```python
from build123d import *

# Parameters (mm, degrees)
BOSS_EXTRUDE1_DEPTH     = 150
BOSS_EXTRUDE2_DEPTH     = 150
SKETCH6_W               = 164.867200615
SKETCH6_H               = 10
BOSS_EXTRUDE4_DEPTH     = 107
BOSS_EXTRUDE5_DEPTH     = 10
BOSS_EXTRUDE6_DEPTH     = 10
SKETCH9_W               = 20
SKETCH9_H               = 170
SKETCH9_R               = 5
BOSS_EXTRUDE7_DEPTH     = 10
CUT_EXTRUDE2_DEPTH      = 281.132270411
CUT_EXTRUDE2_DEPTH_BACK = 281.132270411
CUT_EXTRUDE3_DEPTH      = 263.34809014
CUT_EXTRUDE3_DEPTH_BACK = 263.34809014


with BuildPart() as part:
    # Sketch2 → Boss-Extrude1 (new body)
    with BuildSketch(Plane.XY):
        Polygon((0, 0), (-97, 0), (-97, 107), (0, 10), align=None)
    extrude(amount=BOSS_EXTRUDE1_DEPTH)

    # Sketch4 → Boss-Extrude2 (add)
    with BuildSketch(Plane.XY.offset(150)):
        Polygon((-14.566399692, 24.566399692), (67.867200615, 107), (67.867200615, 0), (0, 0), (0, 10), align=None)
    extrude(amount=-BOSS_EXTRUDE2_DEPTH)

    # Sketch6 → Boss-Extrude4 (add)
    with BuildSketch(Plane(origin=(0, 0, 0), x_dir=(1, 0, 0), z_dir=(0, 1, 0))):
        with Locations((-14.566399692, -155)):
            Rectangle(SKETCH6_W, SKETCH6_H)
        with Locations((-14.566399692, 5)):
            Rectangle(SKETCH6_W, SKETCH6_H)
    extrude(amount=BOSS_EXTRUDE4_DEPTH)

    # Sketch7 → Boss-Extrude5 (add)
    with BuildSketch(Plane.XY.offset(160)):
        Polygon((-97, 107), (-14.566399692, 189.433600308), (67.867200615, 107), align=None)
    extrude(amount=-BOSS_EXTRUDE5_DEPTH)

    # Sketch8 → Boss-Extrude6 (add)
    with BuildSketch(Plane(origin=(0, 0, -10), x_dir=(-1, 0, 0), z_dir=(0, 0, -1))):
        Polygon((-67.867200615, 107), (97, 107), (14.566399692, 189.433600308), align=None)
    extrude(amount=-BOSS_EXTRUDE6_DEPTH)

    # Sketch9 → Boss-Extrude7 (add)
    # profile 1 of 2: a face of its own
    with BuildSketch(Plane(origin=(0, 0, 0), x_dir=(1, 0, 0), z_dir=(0, 1, 0))):
        with Locations((-107, -75)):
            Rectangle(SKETCH9_W, SKETCH9_H)
        with Locations(Location((-107, -145, 0), (0, 0, 270))):
            Circle(SKETCH9_R, mode=Mode.SUBTRACT)
        with Locations(Location((-107, -5, 0), (0, 0, 270))):
            Circle(SKETCH9_R, mode=Mode.SUBTRACT)
    # profile 2 of 2: a face of its own
    with BuildSketch(Plane(origin=(0, 0, 0), x_dir=(1, 0, 0), z_dir=(0, 1, 0))):
        with Locations((77.867200615, -75)):
            Rectangle(SKETCH9_W, SKETCH9_H)
        with Locations(Location((77.867200615, -145, 0), (0, 0, 90))):
            Circle(SKETCH9_R, mode=Mode.SUBTRACT)
        with Locations(Location((77.867200615, -5, 0), (0, 0, 90))):
            Circle(SKETCH9_R, mode=Mode.SUBTRACT)
    extrude(amount=BOSS_EXTRUDE7_DEPTH)

    # Sketch12 → Cut-Extrude2 (cut, two sides: drawn at the far end of the back side and taken through both)
    with BuildSketch(Plane.XY.offset(160).offset(-CUT_EXTRUDE2_DEPTH_BACK)):
        Polygon((-42.02, 161.98), (12.887200615, 161.98), (-14.566399692, 189.433600308), align=None)
    extrude(amount=CUT_EXTRUDE2_DEPTH + CUT_EXTRUDE2_DEPTH_BACK, mode=Mode.SUBTRACT)

    # Sketch14 → Cut-Extrude3 (cut, two sides: drawn at the far end of the back side and taken through both)
    with BuildSketch(Plane.XY.offset(160).offset(-CUT_EXTRUDE3_DEPTH_BACK)):
        Polygon((-14.566399692, 161.98), (67.867200615, 79.546399692), (67.867200615, 107), (12.887200615, 161.98), align=None)
    extrude(amount=CUT_EXTRUDE3_DEPTH + CUT_EXTRUDE3_DEPTH_BACK, mode=Mode.SUBTRACT)


solid = part.part
```
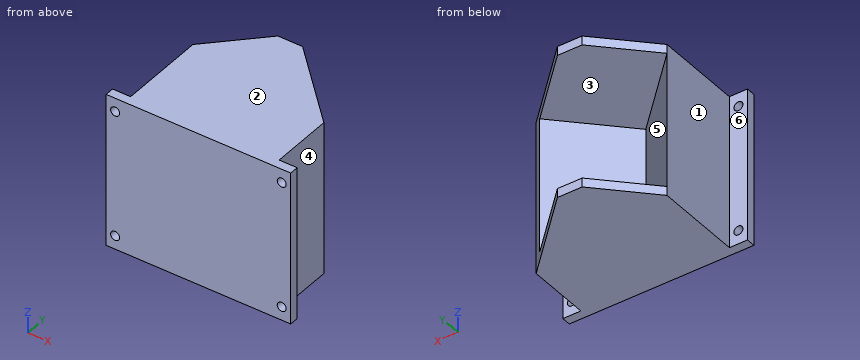
Can you work these out from the model? Positions are in its coordinate system, mm. Face numbers are marked on the shaded views. A direction names the side the tool comes from. Give positions to 0.01 mm unless a question says otherwise; leave off trailing zeros. Loops run counter-clockwise (first coordinate to the right, second up) from the corner with the lowest first, then second, coordinate; pieces in that order, holes last. Notation, with made-up numbers: M 53,45.5 L 64,45.5 A10 ccw 64,51.5 Z; hole C 80.5,-3 d1. An arc over 180 degrees is marked long. Answer in a Markdown table with one row per item.
1. Which directions (+Z, -Z, +X, -X, +Y, -Y) give clear straight access to the entire face, cutting with the end or side of a thin tool? Please do the marked faces 4, 5 and 6.
Taken from the geometry:
| item | result |
|---|---|
| face 4 | +Z, -Z, +X, +Y |
| face 5 | +Y |
| face 6 | +Z, -Z, -X, +Y |
2. Suppose I cut it at A-A on z = 5. Write out the boundary of the cut face in (x, y).
Taken from the geometry:
| item | result |
|---|---|
| outline | M -117,0 L -112,0 L -112,10 L -117,10 Z; M -102,0 L 72.87,0 L 72.87,10 L 67.87,10 L 67.87,79.55 L 54.14,93.27 L -14.57,24.57 L -97,107 L -97,10 L -102,10 Z; M 82.87,0 L 87.87,0 L 87.87,10 L 82.87,10 Z |
3. If I drill on line 1 along X through (y, z) = (6, 5); line 2 along Z through (x, y) = (-26.5, 101.5); line 3 along Y through (x, z) = (-101, 68), over which ranges is the centre line in solid material (lowest first)?
Taken from the geometry:
| item | result |
|---|---|
| line 1 | x = -117 to -112, -102 to 72.87, 82.87 to 87.87 |
| line 2 | z = -10 to 0, 150 to 160 |
| line 3 | y = 0 to 10 |
4. For pin 1 Ø5 at (x, z) = (-89.5, 25.5) entering from +Y; pin 2 Ø6 at (x, z) = (-105, 117.5) entering from +Y; pin 3 Ø3 at (y, z) = (22.5, 67) entering from -X; pin 4 Ø6 at (x, z) = (-107, 145) entering from -Y, each with a flat end and sliding along its axis, tell me the tip position at first contact or that it passes through.
Taken from the geometry:
| item | result |
|---|---|
| pin 1 | stops at y = 102 |
| pin 2 | stops at y = 10 |
| pin 3 | stops at x = -97 |
| pin 4 | passes through |
5. Suppose I cut it at D-D on z = 119. Write out the boundary of the cut face in (x, y).
Taken from the geometry:
| item | result |
|---|---|
| outline | M -117,0 L 87.87,0 L 87.87,10 L 67.87,10 L 67.87,79.55 L 54.14,93.27 L -14.57,24.57 L -97,107 L -97,10 L -117,10 Z |
6. Thinking about a two-plate mould opening in Z: for the marked faces 1, 2 and 3, which applies, released by +Z, released by -Z, zero draft, split by the parting line, or undercut?
Taken from the geometry:
| item | result |
|---|---|
| face 1 | zero draft |
| face 2 | released by +Z |
| face 3 | undercut |
7. Suppose I cut it at B-B on x = -107. Write out the boundary of the cut face in (y, z).
Taken from the geometry:
| item | result |
|---|---|
| outline | M 0,-10 L 10,-10 L 10,0 L 0,0 Z; M 0,10 L 10,10 L 10,140 L 0,140 Z; M 0,150 L 10,150 L 10,160 L 0,160 Z |
8. Suppose I cut it at C-C on y = 139. Write out the boundary of the cut face in (x, z).
Taken from the geometry:
| item | result |
|---|---|
| outline | M -65,-10 L 8.41,-10 L 8.41,0 L -65,0 Z; M -65,150 L 8.41,150 L 8.41,160 L -65,160 Z |
